Geometry check sheet. Reference: the model listing, model coordinates, mm. Face numbers are marked on the shaded views. A direction names the side the tool comes from. Give positions to 0.01 mm unless a question says otherwise; leave off trailing zeros. Loops run counter-clockwise (first coordinate to the right, second up) from the corner with the lowest first, then second, coordinate; pieces in that order, holes last. Notation, with made-up numbers: (-9.5, 17.25) -> (37.5, 17.25) arc R29 ccw to (37.5, 51.25) -> close; hole circle Ø3 at (-38.75, -25.75). An arc over 180 degrees is marked (long way). One line per item, written item: value. Start each with the question number.
(1) Draft check along Y on the marked faces 4, 5 and 6. Enter one of: pulls with the +Y half, pulls with the -Y half, needs draft (parallel to the pull), parting line crosses it, or undercut.
(2) Sectioned sample at A-A, the plane z = 24. Record the cut outline in (x, y), then the cut area to 3 significant figures.
(3) Tool access check on the marked faces 1, 2 and 3. Record the directions out of +Z, -Z, +X, -X, +Y, -Y that give a thin tool (end or side, any length) a straight path to the whole face; none if there is none.
(4) Gauge pin test, flat ends, axial feed: pin 1 Ø10 at (y, z) = (-19.5, 21.5) entering from +X; pin 2 Ø8 at (y, z) = (-1, 24.5) entering from -X; pin 3 Ø11 at (y, z) = (-2.5, 24) entering from +X. Record the tip position at first contact, or that the pin passes through.
(5) Scan lines: line 1 along Y through (x, z) = (11, 1.1); line 2 along Y through (x, z) = (-44, 16); line 3 along X through (y, z) = (3.5, 5.5). Record each from-to range of solid material in increasing order. Write a range as from..to.
(6) Sectioned sample at C-C, the plane x = -23. Record the cut outline in (y, z).
(7) Sectioned sample at B-B, the plane z = 14.5. Record the cut outline in (x, y), then the cut area to 3 significant figures.
(8) Sectioned sample at D-D, the plane y = 23.5. Record the cut outline in (x, z), then the cut area to 3 significant figures.
Autodesk Inventor part; units mm, degrees
ref_plane "Work Plane1" through (12.092, -5.5, 31) normal (0, 0, 1) x (1, 0, 0)
ref_plane "YZ Plane" through (0, 0, 0) normal (1, 0, 0) x (0, 1, 0)
ref_plane "XZ Plane" through (0, 0, 0) normal (0, 1, 0) x (-1, 0, 0)
sketch "Sketch1" plane through (0, 0, 0) normal (0, 0, 1) x (1, 0, 0)
  line L0 (47.7059, -35) -> (-50, -35)
  line L1 (-50, -35) -> (-50, 35)
  line L2 (-50, 35) -> (47.7059, 35)
  line L3 (47.7059, 35) -> (47.7059, -35)
  line L4 (53, -38) -> (53, 38)
  line L5 (53, 38) -> (-53, 38)
  line L6 (-53, 38) -> (-53, -38)
  line L7 (-53, -38) -> (53, -38)
  point P0 (0, 0)
extrude "Extrusion1" add sketch "Sketch1" along normal blind 2 contours L0 L1 L2 L3 | L7 L6 L5 L4
sketch "Sketch2" plane through (-53, 38, 0) normal (0, 1, 0) x (1, 0, 0)
  line L0 (106, 0) -> (130.7184, 17)
  line L1 (106, 0) -> (106, -2)
  line L2 (106, 0) -> (103.092, -2)
  line L3 (106, -2) -> (0, -2)
  line L4 (103.092, -2) -> (106, -2)
  point P0 (53, 0)
extrude "Extrusion2" cut sketch "Sketch2" against normal through all
sketch "Sketch3" plane through (0, 0, 2) normal (0, 0, 1) x (1, 0, 0)
  line L0 (50.092, -38) -> (50.092, 38)
  line L1 (50.092, 38) -> (-53, 38)
  line L2 (-53, 38) -> (-53, -38)
  line L3 (-53, -38) -> (50.092, -38)
  line L4 (-53, -38) -> (-3, -38)
  line L5 (-3, -38) -> (-3, 38)
  line L6 (-3, 38) -> (-53, 38)
  line L7 (-53, 38) -> (-53, -38)
  line L8 (-53, 38) -> (-53, -38)
  line L9 (-53, -38) -> (50.092, -38)
  line L10 (50.092, 38) -> (-53, 38)
  line L11 (-50, -35) -> (-6, -35)
  line L12 (-6, -35) -> (-6, 35)
  line L13 (-6, 35) -> (-50, 35)
  line L14 (-50, 35) -> (-50, -35)
  point P0 (0, 0)
  dimension "d4" = 50
  dimension "d5" = 3
  dimension "d6" = 3
  dimension "d7" = 3
  dimension "d8" = 3
extrude "Extrusion3" add sketch "Sketch3" along normal blind 17 contours L3 L2 L1 L5
sketch3d "3D Sketch1"
sketch "Sketch4" plane through (-3, -38, 2) normal (1, 0, 0) x (0, 0, -1)
  line L0 (0, 76) -> (0, 0)
  line L1 (0, 76) -> (-17, 76)
  line L2 (-17, 0) -> (-17, 76)
  line L3 (0, 0) -> (-17, 0)
  line L4 (-17, 0) -> (-17, 76)
  line L5 (-17, 0) -> (0, 25)
  line L6 (0, 3) -> (0, 73)
  line L7 (-17, 76) -> (0, 51)
  point P0 (2, 38)
  dimension "d11" = 25
  dimension "d12" = 25
loft "Loft1" add profiles "Sketch4" section 2 point at (50.092, -38, 2) contours L5 L0 L3
loft "Loft2" add profiles "Sketch4" section 2 point at (50.092, 38, 2) contours L0 L7 L1
sketch "Sketch6" plane through (0, 0, 2) normal (0, 0, 1) x (1, 0, 0)
  line L0 (11.092, -6.5) -> (35.092, -6.5)
  line L1 (35.092, -6.5) -> (35.092, 6.5)
  line L2 (35.092, 6.5) -> (11.092, 6.5)
  line L3 (11.092, 6.5) -> (11.092, -6.5)
  line L4 (50.092, -38) -> (50.092, 38) construction
  line L5 (50.092, 38) -> (35.092, 6.5) construction
  line L6 (50.092, -38) -> (35.092, -6.5) construction
  line L7 (11.092, -6.5) -> (35.092, 6.5) construction
  line L8 (11.092, 6.5) -> (35.092, -6.5) construction
  line L9 (5.092, -8.5) -> (41.092, -8.5)
  line L10 (41.092, -8.5) -> (41.092, 8.5)
  line L11 (41.092, 8.5) -> (5.092, 8.5)
  line L12 (5.092, 8.5) -> (5.092, -8.5)
  point P0 (0, 0)
  point P1 (23.092, 0)
  dimension "d25" = 24
  dimension "d26" = 13
  dimension "d27" = 15
  dimension "d31" = 6
  dimension "d32" = 6
  dimension "d33" = 2
  dimension "d34" = 2
extrude "Extrusion5" add sketch "Sketch6" along normal blind 19
sketch "Sketch7" plane through (0, 0, 2) normal (0, 0, 1) x (1, 0, 0)
  circle A0 centre (17.592, 0) radius 0.6
  arc A1 (31.1474, 8.5) -> (31.1474, -8.5) centre (17.592, 0) ccw
  line L0 (31.1474, -8.5) -> (5.092, -8.5)
  line L1 (5.092, -8.5) -> (5.092, 8.5)
  line L2 (5.092, 8.5) -> (31.1474, 8.5)
  line L3 (5.092, -8.5) -> (5.092, 8.5)
  line L4 (41.092, -8.5) -> (5.092, -8.5)
  line L5 (5.092, 8.5) -> (41.092, 8.5)
  point P0 (0, 0)
  dimension "d35" = 32
extrude "Extrusion6" add sketch "Sketch7" along normal blind 19 contours L2 L1 L0 A1
sketch "Sketch8" plane through (0, 0, 21) normal (0, 0, 1) x (1, 0, 0)
  line L0 (6.592, -1.125) -> (6.592, -6.2)
  line L1 (6.592, 6.2) -> (6.592, 1.125)
  line L2 (11.092, 6.5) -> (35.092, 6.5)
  line L3 (35.092, -6.5) -> (11.092, -6.5)
  line L4 (39.592, 6.2) -> (39.592, 1.125)
  line L5 (39.592, -1.125) -> (39.592, -6.2)
  line L6 (6.092, -6.5) -> (40.092, -6.5)
  line L7 (40.092, -6.5) -> (40.092, 6.5)
  line L8 (40.092, 6.5) -> (6.092, 6.5)
  line L9 (6.092, 6.5) -> (6.092, -6.5)
  arc A0 (31.1474, 8.5) -> (31.1474, -8.5) centre (17.592, 0) ccw
  line L10 (31.1474, -8.5) -> (41.092, -8.5)
  line L11 (41.092, 8.5) -> (31.1474, 8.5)
  line L12 (41.092, -8.5) -> (41.092, 8.5)
  point P0 (0, 0)
  dimension "d38" = 0.5
  dimension "d39" = 0.5
ref_plane "Work Plane1" through (12.092, -5.5, 31) normal (0, 0, 1) x (1, 0, 0)
extrude "Extrusion7" add sketch "Sketch8" along normal up to surface (10 mm away)
sketch "Sketch9" plane through (0, 0, 21) normal (0, 0, 1) x (1, 0, 0)
  arc A0 (8.4305, -0.75) -> (8.4305, 0.75) centre (9.092, 0) ccw
  arc A1 (37.7534, 0.75) -> (37.7534, -0.75) centre (37.092, 0) ccw
  point P0 (0, 0)
hole "Hole1" at (9.092, 0, 21) at (37.092, 0, 21) direction (0, 0, -1) diameter 1 depth 5 tip angle 118
sketch "Sketch10" plane through (0, 0, 2) normal (0, 0, 1) x (1, 0, 0)
  line L0 (7.592, -4.5) -> (11.092, -4.5)
  line L1 (11.092, -4.5) -> (11.092, 4.5)
  line L2 (11.092, 4.5) -> (7.592, 4.5)
  line L3 (7.592, 4.5) -> (7.592, -4.5)
  line L4 (11.092, 6.5) -> (11.092, -6.5)
  line L5 (35.092, 6.5) -> (11.092, 6.5) construction
  line L6 (11.092, 6.5) -> (7.592, 4.5) construction
  line L7 (7.592, -4.5) -> (11.092, -6.5) construction
  point P0 (0, 0)
  dimension "d49" = 3.5
  dimension "d50" = 9
extrude "Extrusion8" cut sketch "Sketch10" along normal blind 14 and the other way blind 3
sketch "Sketch11" plane through (0, 0, 0) normal (0, 0, -1) x (-1, 0, 0)
  circle A0 centre (-44.7059, -33) radius 2.125
  circle A1 centre (-44.7059, 33) radius 2.125
  circle A2 centre (48, -10) radius 2.125
  circle A3 centre (48, 10) radius 2.125
  point P0 (0, 0)
extrude "Extrusion9" cut sketch "Sketch11" against normal through all
sketch "Sketch12" plane through (0, 0, 2) normal (0, 0, 1) x (1, 0, 0)
  circle A0 centre (44.7059, -33) radius 2.125
  circle A1 centre (44.7059, 33) radius 2.125
  arc A2 (-50, -10.7181) -> (-50, -9.2819) centre (-48, -10) ccw
  arc A3 (-50, 9.2819) -> (-50, 10.7181) centre (-48, 10) ccw
  circle A4 centre (44.7059, -33) radius 4
  circle A5 centre (44.7059, 33) radius 4
  circle A6 centre (-48, -10) radius 2.125
  circle A7 centre (-48, -10) radius 4
  circle A8 centre (-48, 10) radius 2.125
  circle A9 centre (-48, 10) radius 4
  point P0 (0, 0)
  dimension "d57" = 8
  dimension "d58" = 8
  dimension "d59" = 8
  dimension "d60" = 8
extrude "Extrusion10" cut sketch "Sketch12" along normal through all contours A0 | A1 | A6 A2 | A8 A3 | A4 | A5 | A7 | A9
sketch "Sketch15" plane through (0, 0, 2) normal (0, 0, 1) x (1, 0, 0)
  line L0 (-45, -6.5) -> (-35, -6.5)
  line L1 (-35, -6.5) -> (-35, 6.5)
  line L2 (-35, 6.5) -> (-45, 6.5)
  line L3 (-45, 6.5) -> (-45, -6.5)
  line L4 (-50, -35) -> (-50, -13.4641) construction
  line L5 (-50, -35) -> (-45, -6.5) construction
  line L6 (-50, 35) -> (-6, 35) construction
  line L7 (-45, 6.5) -> (-50, 35) construction
  line L8 (-50, -6.5359) -> (-50, 6.5359) construction
  circle A0 centre (11, -17) radius 2
  line L9 (-3, -38) -> (-3, 38)
  line L10 (-3, -38) -> (50.092, -38)
  point P0 (0, 0)
  dimension "d73" = 10
  dimension "d74" = 13
  dimension "d75" = 5
  dimension "d76" = 4
  dimension "d77" = 14
  dimension "d78" = 21
extrude "Extrusion12" cut sketch "Sketch15" against normal through all
equation "\"d6\" = d5"
equation "\"d7\" = d5"
equation "\"d8\" = d5"
equation "\"d12\" = d11"
equation "\"d32\" = d31"
equation "\"d34\" = d33"
equation "\"d39\" = d38"
properties part number "cover" material "Ogólne"
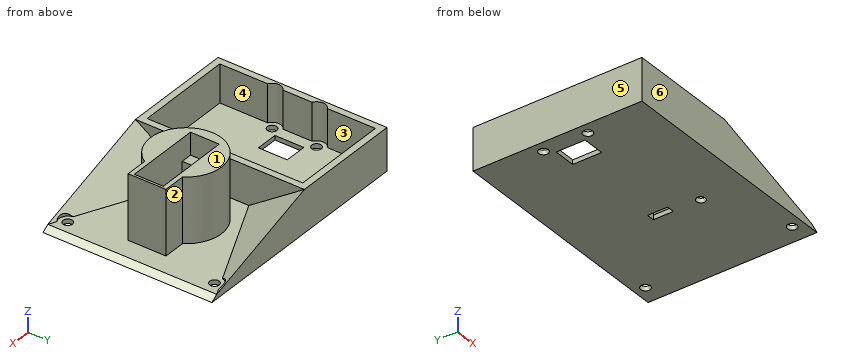
Calculated:
1. face 4: undercut
1. face 5: needs draft
1. face 6: pulls with the -Y half
2. outline: (31.15, -8.5) -> (41.09, -8.5) -> (41.09, 8.5) -> (31.15, 8.5) arc R16 ccw (long way) to start; hole (6.09, -6.5) -> (40.09, -6.5) -> (40.09, 6.5) -> (6.09, 6.5) -> close
2. area: 503 mm2
3. face 1: +Z, +X, -X, +Y, -Y
3. face 2: +Z, +X
3. face 3: +Z
4. pin 1: stops at x = 24.36
4. pin 2: stops at x = 1.59
4. pin 3: stops at x = 41.09
5. line 1: y = -38..-19, -15..-4.5, 4.5..38
5. line 2: y = -38..-35, 35..38
5. line 3: x = -53..-50, -6..-3, 1.98..7.59, 35.09..41.09
6. outline: (-38, 0) -> (38, 0) -> (38, 19) -> (35, 19) -> (35, 2) -> (-35, 2) -> (-35, 19) -> (-38, 19) -> close
7. outline: (-53, -38) -> (11.05, -38) -> (-3, -31.38) -> (-3, 31.38) -> (11.05, 38) -> (-53, 38) -> close; (31.15, -8.5) -> (41.09, -8.5) -> (41.09, 8.5) -> (31.15, 8.5) arc R16 ccw (long way) to start; hole (-50, -35) -> (-6, -35) -> (-6, 35) -> (-50, 35) -> (-50, 13.46) arc R4 ccw to (-50, 6.54) -> (-50, -6.54) arc R4 ccw to (-50, -13.46) -> close; hole (7.59, -4.5) -> (11.09, -4.5) -> (11.09, -6.5) -> (35.09, -6.5) -> (35.09, 6.5) -> (11.09, 6.5) -> (11.09, 4.5) -> (7.59, 4.5) -> close
7. area: 1,390 mm2
8. outline: (-53, 0) -> (53, 0) -> (50.09, 2) -> (19.3, 2) -> (-3, 9.14) -> (-3, 19) -> (-6, 19) -> (-6, 2) -> (-50, 2) -> (-50, 19) -> (-53, 19) -> close
8. area: 391 mm2
